Here's how the part is built. I have some questions about the finished solid (model axes, mm). Face numbers are marked on the shaded views. A direction names the side the tool comes from. Round coordinates to 2 decimals unless told otherwise and drop trailing zeros. Order: outer loops, then holes, each group sorted by start corner. A loop starts at its lowest first (then second) coordinate and runs counter-clockwise, first axis right, second up. Notation, with made-up numbers: (61, -7) - (95, -7) arc R15 ccw to (95, 4) - close; hole circle Ø9 at (72, -39.75). An arc over 180 degrees is marked (long way). Answer as a JSON object with one key per item and string values.
```python
from build123d import *

# Parameters (mm, degrees)
PAD_DEPTH    = 10
SKETCH001_W  = 10
SKETCH001_H  = 23
PAD001_DEPTH = 3
SKETCH002_W  = 10
SKETCH002_H  = 3
PAD002_DEPTH = 30
FILLET_R     = 4.49
FILLET001_R  = 1
FILLET002_R  = 2


with BuildPart() as part:
    # Sketch → Pad (new body)
    with BuildSketch(Plane.XZ):
        with BuildLine():
            ThreePointArc((3.68273, 0), (0, 7.75), (-3.68273, 0))
            Line((-3.68273, 0), (3.68273, 0))
        make_face()
    extrude(amount=PAD_DEPTH)

    # Sketch001 → Pad001 (join)
    with BuildSketch(Plane.XY):
        with Locations((0, 11.5)):
            Rectangle(SKETCH001_W, SKETCH001_H)
    extrude(amount=PAD001_DEPTH)

    # Sketch002 (on Face7 of Pad001) → Pad002 (join)
    with BuildSketch(Plane(origin=(0, 0, 3), x_dir=(-1, 0, 0), z_dir=(0, 0, 1))):
        with Locations((0, -21.5)):
            Rectangle(SKETCH002_W, SKETCH002_H)
    extrude(amount=PAD002_DEPTH)

    # Fillet
    fillet_edges = [part.edges().sort_by_distance(p)[0] for p in [
        (0, 20, 3),
        (0, 0, 3),
    ]]
    fillet(fillet_edges, radius=FILLET_R)

    # Fillet001
    fillet001_edges = [part.edges().sort_by_distance(p)[0] for p in [
        (5, 21.5, 33),
        (0, 23, 33),
        (-5, 21.5, 33),
        (0, 20, 33),
    ]]
    fillet(fillet001_edges, radius=FILLET001_R)

    # Fillet002
    fillet002_edges = [part.edges().sort_by_distance(p)[0] for p in [
        (0, -10, 0),
        (0, -10, 7.75),
    ]]
    fillet(fillet002_edges, radius=FILLET002_R)


solid = part.part
```
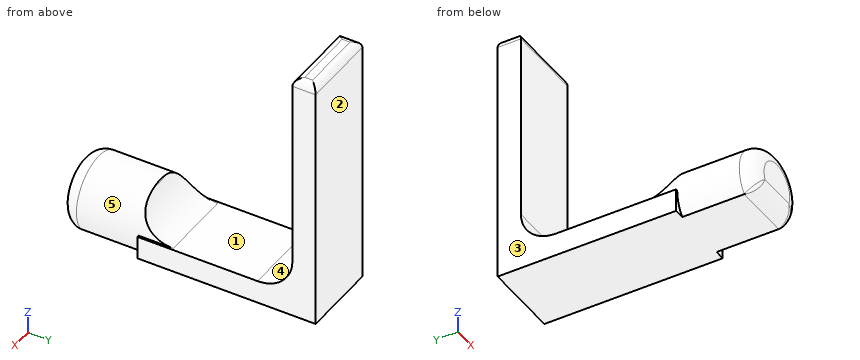
1. For the marked faces 4 and 5, which set-ups out of +Z, -Z, +X, -X, +Y, -Y let a thin tool reach every point of the face, with its end or its side?
Responses:
{"face 4": "+Z, +X, -X", "face 5": "-Y"}
2. Imagine slicing it at A-A (x = 0). List the corners of the cut face in (y, z) for me.
Responses:
{"outline": "(-10, 2) arc R2 ccw to (-8, 0) - (23, 0) - (23, 32) arc R1 ccw to (22, 33) - (21, 33) arc R1 ccw to (20, 32) - (20, 7.49) arc R4.49 cw to (15.51, 3) - (4.49, 3) arc R4.49 cw to (0, 7.49) - (0, 7.75) - (-8, 7.75) arc R2 ccw to (-10, 5.75) - close"}
3. For P1, Ø10, axis at y = 11, z = 13.5, coming from the +X side; P2, Ø2, axis at x = -1.5, z = 25, coming from the -Y side; P3, Ø4, axis at x = -1.5, y = 2.5, coming from the +Z side; P4, Ø5, axis at x = -3, y = 3.5, coming from the +Z side, each with a flat end and sliding along its axis, tell me the tip position at first contact or that it passes through.
Responses:
{"P1": "through", "P2": "y = 20", "P3": "z = 5.43", "P4": "z = 4.67"}
4. Thinking about a two-plate mould opening in Y: for the marked faces 1, 2 and 3, which applies, pulls with the +Y half, pulls with the -Y half, needs draft (parallel to the pull), parting line crosses it, or undercut?
Responses:
{"face 1": "undercut", "face 2": "pulls with the +Y half", "face 3": "needs draft"}
5. Imagine slicing it at B-B (y = 12). List the corners of the cut face in (x, z) for me, plus the area to 3 significant figures.
Responses:
{"outline": "(-5, 0) - (5, 0) - (5, 3) - (-5, 3) - close", "area": "30.0 mm2"}
6. If I drill on L1, parallel to Y at x = -3.5, z = 25.5; L2, parallel to Z at x = -0.25, y = -4; L3, parallel to Z at x = -2.25, y = 5, over which ranges is the centre line in solid material (lowest first)? Write a range as [from, to].
Responses:
{"L1": "[20, 23]", "L2": "[0, 7.74]", "L3": "[0, 3]"}
7. Imagine slicing it at D-D (y = -1). List the corners of the cut face in (x, z) for me.
Responses:
{"outline": "(-3.68, 0) - (3.68, 0) arc R4.75 ccw (long way) to start"}
8. Imagine slicing it at C-C (z = 21.5). List the corners of the cut face in (x, y) for me.
Responses:
{"outline": "(-5, 20) - (5, 20) - (5, 23) - (-5, 23) - close"}
